For this review, take the finished solid that the model builds, in its own axes (mm). Face numbers are marked on the shaded views. A direction names the side the tool comes from. Coordinates: 2 decimals unless noted, no trailing zeros. Loops run counter-clockwise (first coordinate to the right, second up) from the corner with the lowest first, then second, coordinate; pieces in that order, holes last. Notation, with made-up numbers: M 1,15 L 47,15 A18 cw 47,50 Z; hole C 26,27.25 d4. An arc over 180 degrees is marked long. Write item = value, one per line.
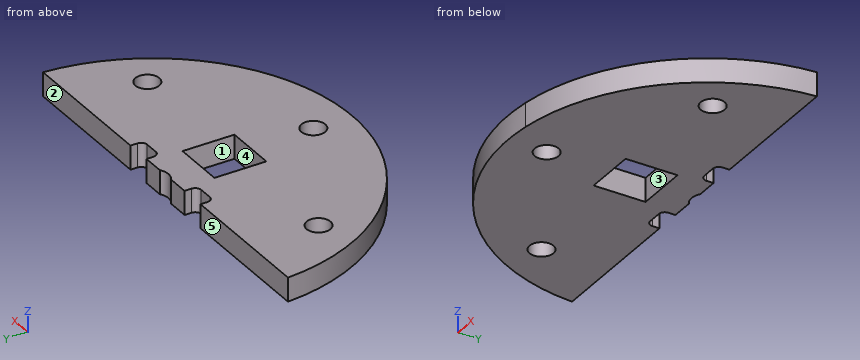
from build123d import *

# Parameters (mm, degrees)
MODEL_R                 = 1.5
MODEL_W                 = 6.5
MODEL_H                 = 6.5
SALIENTE_EXTRUIR1_DEPTH = 3


with BuildPart() as part:
    # Model → Saliente-Extruir1 (new body)
    with BuildSketch(Plane.XY):
        with BuildLine():
            Line((191.396871733, 188.964281637), (194.105949351, 188.964281637))
            Line((194.105949351, 188.964281637), (194.105949351, 188.089281637))
            ThreePointArc((194.105949351, 188.089281637), (194.325619265, 187.558951551), (194.855949351, 187.339281637))
            Line((194.855949351, 187.339281637), (196.605949351, 187.339281637))
            ThreePointArc((196.605949351, 187.339281637), (197.136279437, 187.558951551), (197.355949351, 188.089281637))
            Line((197.355949351, 188.089281637), (197.355949351, 188.964281637))
            Line((197.355949351, 188.964281637), (215.17808095, 188.964281637))
            ThreePointArc((215.17808095, 188.964281637), (208.476468276, 173.498317967), (193.480949351, 165.80143179))
            ThreePointArc((193.480949351, 165.80143179), (174.362087289, 171.27143453), (165.283817753, 188.964281637))
            Line((165.283817753, 188.964281637), (183.105949351, 188.964281637))
            Line((183.105949351, 188.964281637), (183.105949351, 188.089281637))
            ThreePointArc((183.105949351, 188.089281637), (183.325619265, 187.558951551), (183.855949351, 187.339281637))
            Line((183.855949351, 187.339281637), (185.605949351, 187.339281637))
            ThreePointArc((185.605949351, 187.339281637), (186.136279437, 187.558951551), (186.355949351, 188.089281637))
            Line((186.355949351, 188.089281637), (186.355949351, 188.964281637))
            Line((186.355949351, 188.964281637), (189.06502697, 188.964281637))
            ThreePointArc((189.06502697, 188.964281637), (190.230949351, 188.589281637), (191.396871733, 188.964281637))
        make_face()
        with Locations((172.802524293, 180.526975738)):
            Circle(MODEL_R, mode=Mode.SUBTRACT)
        with Locations((190.230949351, 170.464669839)):
            Circle(MODEL_R, mode=Mode.SUBTRACT)
        with Locations((207.659374409, 180.526975738)):
            Circle(MODEL_R, mode=Mode.SUBTRACT)
        with Locations((190.230949351, 181.589281637)):
            Rectangle(MODEL_W, MODEL_H, mode=Mode.SUBTRACT)
    extrude(amount=SALIENTE_EXTRUIR1_DEPTH)


solid = part.part
Q1. Machinability: for the marked faces 1 and 2, which of the approach directions +Z, -Z, +X, -X, +Y, -Y give a long, thin tool a straight path to every point of the face, cutting with its end or side? Answer none if there is none.
Solved:
face_1 = +Z, -Z
face_2 = +Z, -Z, +X, -X, +Y
Q2. For line 1 along X through (y, z) = (187.5, 1.85); line 2 along Y through (x, z) = (191, 1.45); line 3 along Y through (x, z) = (187.5, 0.7), list the stretches that pass through material, from the lowest coordinate up.
Solved:
line_1 = 165.42 to 183.39, 186.07 to 194.39, 197.07 to 215.04
line_2 = 165.6 to 169.18, 171.75 to 178.34, 184.84 to 188.74
line_3 = 165.74 to 178.34, 184.84 to 188.96
Q3. Add section C-C (z = 0.8). Write out the cut boundary in (x, y).
Solved:
outline = M 165.28,188.96 A25 ccw 215.18,188.96 L 197.36,188.96 L 197.36,188.09 A0.75 cw 196.61,187.34 L 194.86,187.34 A0.75 cw 194.11,188.09 L 194.11,188.96 L 191.4,188.96 A2 cw 189.07,188.96 L 186.36,188.96 L 186.36,188.09 A0.75 cw 185.61,187.34 L 183.86,187.34 A0.75 cw 183.11,188.09 L 183.11,188.96 Z; hole C 172.8,180.53 d3; hole M 186.98,178.34 L 193.48,178.34 L 193.48,184.84 L 186.98,184.84 Z; hole C 190.23,170.46 d3; hole C 207.66,180.53 d3
Q4. Add section A-A (y = 182.75). Write out the cut boundary in (x, z).
Solved:
outline = M 166.49,0 L 186.98,0 L 186.98,3 L 166.49,3 Z; M 193.48,0 L 213.97,0 L 213.97,3 L 193.48,3 Z
Q5. For pin 1 Ø1.4 at (x, z) = (195.5, 2) entering from +Y; pin 2 Ø0.9 at (y, z) = (180.5, 1.5) entering from -X; pin 3 Ø3.5 at (x, y) = (172.8, 180.53) entering from -Z; pin 4 Ø1 at (x, z) = (184.5, 2.5) entering from -Y, all flat-tipped, find the tip position at first contact; note any pin that passes through.
Solved:
pin_1 = 187.34
pin_2 = 167.16
pin_3 = 0
pin_4 = 166.14
Q6. Add section B-B (x = 188). Write out the cut boundary in (y, z).
Solved:
outline = M 165.69,0 L 178.34,0 L 178.34,3 L 165.69,3 Z; M 184.84,0 L 188.96,0 L 188.96,3 L 184.84,3 Z
Q7. Draft analysis for pull direction X (two halves, no side actions). For the marked faces 3, 4 and 5, state which applies: +X half, -X half, draft (parallel to the pull), parting line (faces both ways), or undercut.
Solved:
face_3 = undercut
face_4 = undercut
face_5 = draft
Q8. Add section D-D (y = 179.5). Write out the cut boundary in (x, z).
Solved:
outline = M 167.82,0 L 171.71,0 L 171.71,3 L 167.82,3 Z; M 173.9,0 L 186.98,0 L 186.98,3 L 173.9,3 Z; M 193.48,0 L 206.57,0 L 206.57,3 L 193.48,3 Z; M 208.75,0 L 212.64,0 L 212.64,3 L 208.75,3 Z
